Could you check a few things on this model? Use its own coordinates, in mm. Coordinates: 2 decimals unless noted, no trailing zeros. Order: outer loops, then holes, each group sorted by start corner. A loop starts at its lowest first (then second) coordinate and runs counter-clockwise, first axis right, second up. Notation, with made-up numbers: (-22, -14.5) - (37, -14.5) arc R21 ccw to (37, -5.5) - close; hole circle Ø8 at (48.25, 7.25). An arc over 180 degrees is marked (long way). Answer as a JSON object with one key per item and string values. Group by question number.
(1) Imagine slicing it at B-B, the plane x = -10.5. Write out the boundary of the cut face in (y, z) (3 decimals).
(2) Please list where these lines run through material, in increasing order: probe 1 along Z at (x, y) = (-4, 0.15); probe 2 along X at (y, z) = (0.45, -18.25); probe 3 along Y at (x, z) = (-2, -0.75).
(3) Imagine slicing it at A-A, the plane y = 0.3. Write out the boundary of the cut face in (x, z).
(4) Imagine slicing it at C-C, the plane z = -17. Write out the boundary of the cut face in (x, y) (3 decimals), and give its area (3 significant figures).
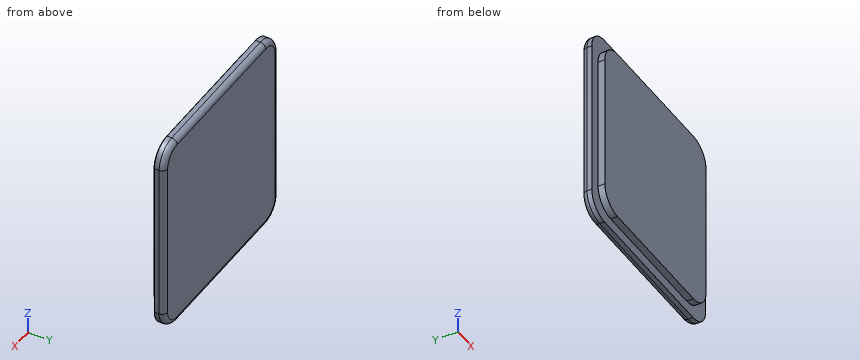
Autodesk Inventor part; units mm, degrees
ref_plane "YZ Plane" through (0, 0, 0) normal (1, 0, 0) x (0, 1, 0)
ref_plane "XZ Plane" through (0, 0, 0) normal (0, 1, 0) x (-1, 0, 0)
ref_plane "XY Plane" through (0, 0, 0) normal (0, 0, 1) x (1, 0, 0)
sketch "Sketch1" plane through (0, 0, 0) normal (0, 1, 0) x (-1, 0, 0)
  line L0 (0, 0) -> (22.86, 0)
  line L1 (22.86, 0) -> (22.86, -24.13)
  line L2 (22.86, -24.13) -> (0, -24.13)
  line L3 (0, -24.13) -> (0, 0)
  dimension "d0" = 24.13
  dimension "d1" = 22.86
extrude "Extrusion1" add sketch "Sketch1" along normal blind 2
sketch "Sketch2" plane through (0, 0, 0) normal (0, -1, 0) x (1, 0, 0)
  line L0 (-1.27, -1.27) -> (-21.59, -1.27)
  line L1 (-21.59, -1.27) -> (-21.59, -22.86)
  line L2 (-21.59, -22.86) -> (-1.27, -22.86)
  line L3 (-1.27, -22.86) -> (-1.27, -1.27)
  line L4 (-22.86, 0) -> (0, 0)
  line L5 (0, -24.13) -> (-22.86, -24.13)
  line L6 (0, 0) -> (0, -24.13)
  line L7 (-22.86, -24.13) -> (-22.86, 0)
  line L8 (0, 0) -> (0, -24.13)
  line L9 (0, 0) -> (-22.86, 0)
  line L10 (-22.86, 0) -> (-22.86, -24.13)
  line L11 (-22.86, -24.13) -> (0, -24.13)
  line L12 (0, -24.13) -> (0, 0)
  dimension "d4" = 20.32
  dimension "d5" = 21.59
  dimension "d6" = 1.27
  dimension "d7" = 1.27
  dimension "d8" = 1.27
  dimension "d9" = 1.27
extrude "Extrusion2" cut sketch "Sketch2" against normal blind 0.8
fillet "Fillet1" radius 2.54 8 edges at (0, 1.4, 0) (0, 1.4, -24.13) (-22.86, 1.4, -24.13) (-22.86, 1.4, 0) (-21.59, 0.4, -1.27) (-1.27, 0.4, -1.27) (-1.27, 0.4, -22.86) (-21.59, 0.4, -22.86)
fillet "Fillet2" radius 0.635 8 edges at (-22.1161, 2, -0.7439) (-11.43, 2, 0) (-0.7439, 2, -0.7439) (0, 2, -12.065) (-0.7439, 2, -23.3861) (-11.43, 2, -24.13) (-22.1161, 2, -23.3861) (-22.86, 2, -12.065)
equation "\"d6\" = d7"
equation "\"d8\" = d9"
properties part number "micro lipo lid"
Result set:
{
 "1": {"outline": "(0, -22.86) - (0.8, -22.86) - (0.8, -24.13) - (1.365, -24.13) arc R0.635 ccw to (2, -23.495) - (2, -0.635) arc R0.635 ccw to (1.365, 0) - (0.8, 0) - (0.8, -1.27) - (0, -1.27) - close"},
 "2": {"probe 1": "z = -22.86 to -1.27", "probe 2": "x = -21.59 to -1.27", "probe 3": "y = 0.8 to 2"},
 "3": {"outline": "(-21.59, -20.32) arc R2.54 ccw to (-19.05, -22.86) - (-3.81, -22.86) arc R2.54 ccw to (-1.27, -20.32) - (-1.27, -3.81) arc R2.54 ccw to (-3.81, -1.27) - (-19.05, -1.27) arc R2.54 ccw to (-21.59, -3.81) - close"},
 "4": {"outline": "(-22.86, 0.8) - (-21.59, 0.8) - (-21.59, 0) - (-1.27, 0) - (-1.27, 0.8) - (0, 0.8) - (0, 1.365) arc R0.635 ccw to (-0.635, 2) - (-22.225, 2) arc R0.635 ccw to (-22.86, 1.365) - close", "area": "43.5 mm^2"}
}
